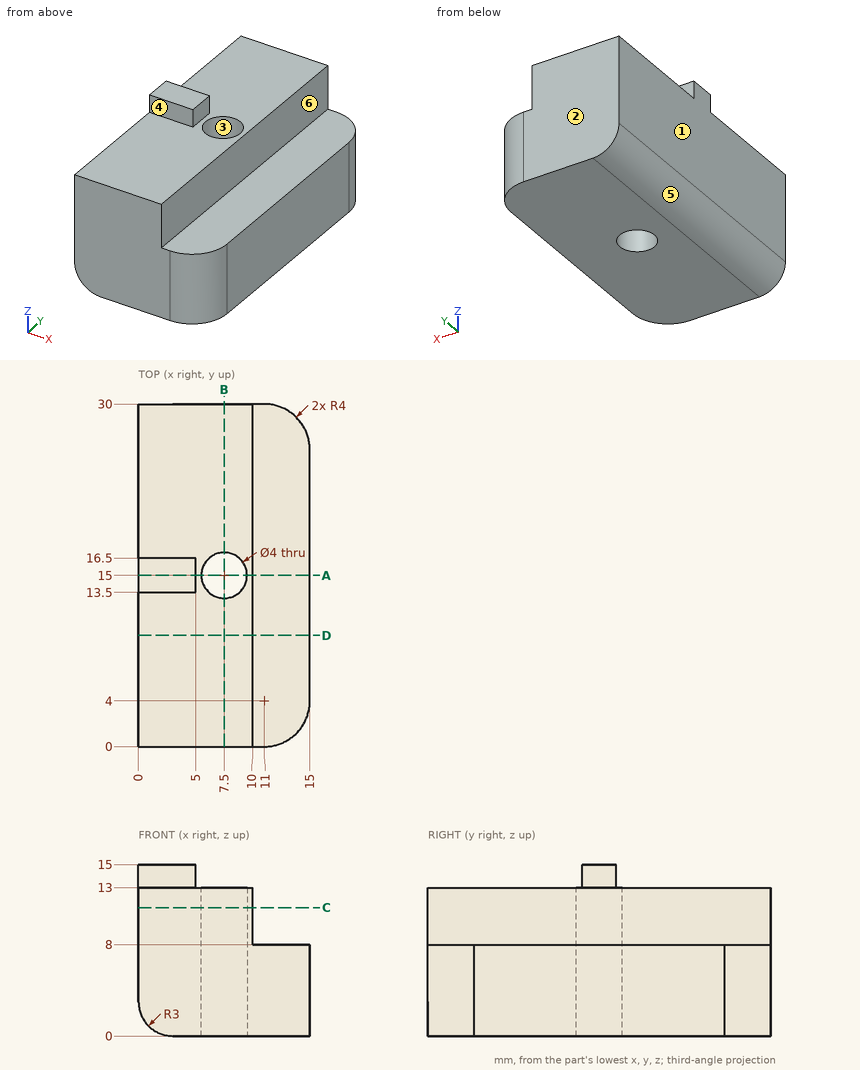
Input: dimensioned drawing with shaded views. Units: mm. Origin: part minimum x, y, z. A direction names the side the tool comes from. Give positions to 0.01 mm unless a question says otherwise; leave off trailing zeros. Write each loop counter-clockwise with the first axis right and the second up, starting at its lowest first coordinate (ties: lowest second). Pieces come first, ordered by that corner, then holes.
Q1. Section C-C, the plane z = 11.25. Output: boundary loops of the cut face in (x, y).
Q2. Section A-A, the plane y = 15. Output: boundary loops of the cut face in (x, z).
Q3. First-contact query: P1, Ø6, axis at x = 9, y = 4, coming from the +Z side; P2, Ø2, axis at y = 26, z = 9.5, coming from the +X side; P3, Ø1.6, axis at x = 3.5, z = 14, coming from the +Y side; P4, Ø1, axis at x = 8, y = 15, coming from the -Z side. Flat tips, straight axial feed; report the tip coordinate or a pass-through.
Q4. Section D-D, the plane y = 9.75. Output: boundary loops of the cut face in (x, z), plus the area to 3 significant figures.
Q5. Section B-B, the plane x = 7.5. Output: boundary loops of the cut face in (y, z), plus the area to 3 significant figures.
Q6. Pull-direction query (X, two-part tool) for the marked faces 1, 2 and 3; classes: pulls with the +X half, pulls with the -X half, needs draft (parallel to the pull), parting line crosses it, or undercut.
Q7. Set-up query: the marked faces 4, 5 and 6. Return all of +Z, -Z, +X, -X, +Y, -Y with unobstructed straight access to the full face (end or side cutting, diameter ignored); none if empty.
Q8. Material intervals for probe 1 along Y at (x, z) = (7.5, 8.25); probe 2 along Z at (x, y) = (5.75, 18.5); probe 3 along Y at (x, z) = (8.75, 9.75), sorted ascending.
Filled in:
1. outline: (0, 0) - (10, 0) - (10, 30) - (0, 30) - close; hole circle Ø4 at (7.5, 15)
2. outline: (0, 3) arc R3 ccw to (3, 0) - (5.5, 0) - (5.5, 13) - (5, 13) - (5, 15) - (0, 15) - close; (9.5, 0) - (15, 0) - (15, 8) - (10, 8) - (10, 13) - (9.5, 13) - close
3. P1: stops at z = 13
3. P2: stops at x = 10
3. P3: stops at y = 16.5
3. P4: passes through
4. outline: (0, 3) arc R3 ccw to (3, 0) - (15, 0) - (15, 8) - (10, 8) - (10, 13) - (0, 13) - close
4. area: 168 mm2
5. outline: (0, 0) - (13, 0) - (13, 13) - (0, 13) - close; (17, 0) - (30, 0) - (30, 13) - (17, 13) - close
5. area: 338 mm2
6. face 1: pulls with the -X half
6. face 2: needs draft
6. face 3: undercut
7. face 4: +Z, +X, -X, -Y
7. face 5: -Z, -X, +Y, -Y
7. face 6: +Z, +X, +Y, -Y
8. probe 1: y = 0 to 13, 17 to 30
8. probe 2: z = 0 to 13
8. probe 3: y = 0 to 13.44, 16.56 to 30
